Geometry: final body of the model. Coordinates: model frame, mm. Face numbers are marked on the shaded views. A direction names the side the tool comes from. Give positions to 0.01 mm unless a question says otherwise; leave off trailing zeros. Order: outer loops, then holes, each group sorted by start corner. A loop starts at its lowest first (then second) coordinate and runs counter-clockwise, first axis right, second up. Notation, with made-up numbers: M -24.5,46 L 5.5,46 A31 cw 5.5,81 Z; hole C 23,-14 d8. An arc over 180 degrees is marked long. Write item = value, one per line. Start each with the question number.
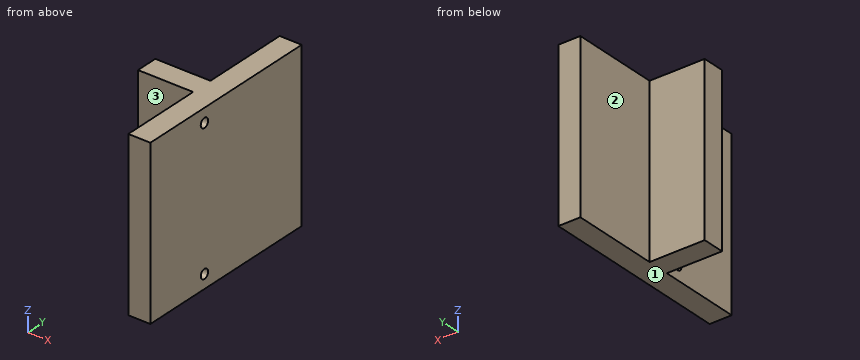
Autodesk Inventor part; units mm, degrees
ref_plane "YZ Plane" through (0, 0, 0) normal (1, 0, 0) x (0, 1, 0)
ref_plane "XZ Plane" through (0, 0, 0) normal (0, 1, 0) x (-1, 0, 0)
ref_plane "XY Plane" through (0, 0, 0) normal (0, 0, 1) x (1, 0, 0)
sketch "Skizze1" plane through (0, 0, 0) normal (0, 0, 1) x (1, 0, 0)
  line L0 (0, 54) -> (0, -44)
  line L1 (-33.6, 0) -> (5.6, 0)
  line L2 (-8, 40) -> (0, 40)
  line L3 (0, 40) -> (0, -30)
  line L4 (0, -30) -> (-8, -30)
  line L5 (-8, -30) -> (-8, 0)
  line L6 (-8, 0) -> (-28, 0)
  line L7 (-28, 0) -> (-28, 8)
  line L8 (-28, 8) -> (-8, 8)
  line L9 (-8, 8) -> (-8, 40)
  point P0 (0, 0)
  dimension "d0" = 70
  dimension "d1" = 8
  dimension "d2" = 20
  dimension "d3" = 8
  dimension "d4" = 40
extrude "Extrusion1" add sketch "Skizze1" along normal mid plane 60
sketch "Skizze2" plane through (0, -30, 30) normal (1, 0, 0) x (0, 0, -1)
  point P0 (30, 30)
sketch "Skizze3" plane through (0, -30, 30) normal (1, 0, 0) x (0, 0, -1)
  line L0 (-12, 30) -> (72, 30)
  line L1 (30, -14) -> (30, 84)
  line L2 (60, 70) -> (0, 70)
  point P0 (30, 30)
  point P1 (5, 25)
  point P2 (55, 25)
  dimension "d7" = 50
  dimension "d8" = 45
hole "Bohrung1" at (0, -5, 25) at (0, -5, -25) direction (-1, 0, 0) diameter 3.4 end through all
properties part number "25_Laser_adapter"
1) Cut plane C-C (z = -25). Return loops of the section in (x, y), plus the area to 3 significant figures.
2) Cut plane A-A (z = 17). Return loops of the section in (x, y).
3) Cut plane B-B (y = -5). Return loops of the section in (x, z).
4) Ray query, L1, parallel to Z at x = -5.25, y = -5; L2, parallel to Y at x = -4.5, z = -25; L3, parallel to X at y = 34.5, z = 4.5. Return the intervals inside material, ascending.
5) Access query for the marked faces 1, 2 and 3. Directions: +Z, -Z, +X, -X, +Y, -Y. A direction counts if a zero-diameter tool reaches every point of the face in a straight line with its end or side. Return the directions, or none.
6) Cut plane D-D (x = -16). Return loops of the section in (y, z), plus the area to 3 significant figures.
7) Pin query (flat end, axial travel): pin 1 Ø1.5 at (x, z) = (-21.5, 4.5) entering from -Y; pin 2 Ø4 at (y, z) = (-13.5, 12.5) entering from -X; pin 3 Ø6 at (x, z) = (-15, -13) entering from +Y. Return the tip coordinate at first contact, or that it passes through.
Reply:
q1.outline = M -28,0 L -8,0 L -8,-3.3 L 0,-3.3 L 0,40 L -8,40 L -8,8 L -28,8 Z; M -8,-30 L 0,-30 L 0,-6.7 L -8,-6.7 Z
q1.area = 693 mm²
q2.outline = M -28,0 L -8,0 L -8,-30 L 0,-30 L 0,40 L -8,40 L -8,8 L -28,8 Z
q3.outline = M -8,-30 L 0,-30 L 0,-26.7 L -8,-26.7 Z; M -8,-23.3 L 0,-23.3 L 0,23.3 L -8,23.3 Z; M -8,26.7 L 0,26.7 L 0,30 L -8,30 Z
q4.L1 = -30 to -26.7, -23.3 to 23.3, 26.7 to 30
q4.L2 = -30 to -6.7, -3.3 to 40
q4.L3 = -8 to 0
q5.face_1 = -Z, +X, -X, +Y, -Y
q5.face_2 = +Z, -Z, -X, +Y
q5.face_3 = +Z, -Z, -X, -Y
q6.outline = M 0,-30 L 8,-30 L 8,30 L 0,30 Z
q6.area = 480 mm²
q7.pin_1 = 0
q7.pin_2 = -8
q7.pin_3 = 8
